For this review, use the dimensioned drawing (mm, ordinates from the lowest corner) and the shaded views. A direction names the side the tool comes from. Round coordinates to 2 decimals unless told otherwise and drop trailing zeros. Write each loop counter-clockwise with the first axis right and the second up, starting at its lowest first coordinate (ties: lowest second). Pieces come first, ordered by that corner, then holes.
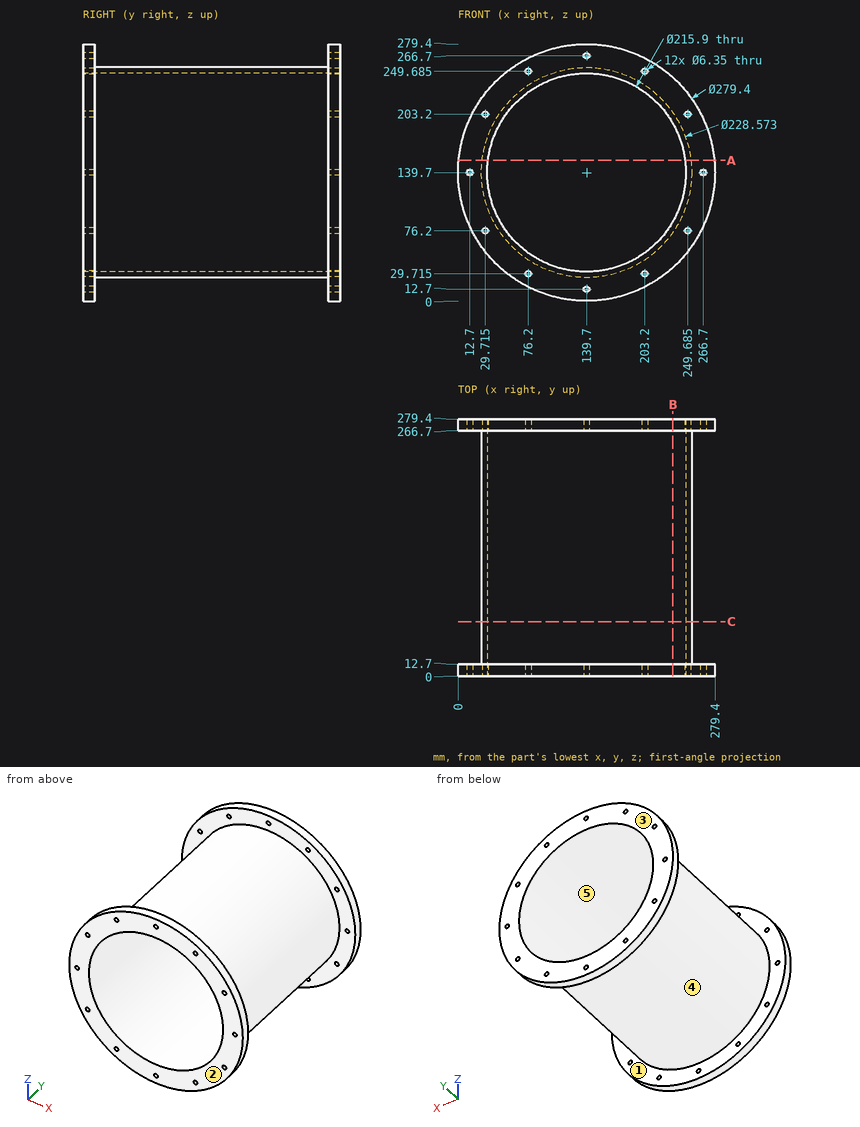
1) The part is to be moulded in two halves that separate along Z. For the marked faces 3, 4 and 5, say which applies: pulls with the +Z half, pulls with the -Z half, needs draft (parallel to the pull), parting line crosses it, or undercut.
2) Add section C-C on y = 59. State the section outline as (x, z) points.
3) For P1, Ø4, axis at x = 12.7, z = 139.7, coming from the +Y side; P2, Ø3, axis at y = 233.5, z = 200.5, coming from the +X side; P3, Ø6, axis at y = 79, z = 35, coming from the +X side; P4, Ø3, axis at x = 205.5, y = 138, coming from the -Z side, all flat-tipped, find the tip position at first contact; note any pin that passes through.
4) For line 1 along Z through (x, y) = (139, 3); line 2 along Y through (x, z) = (196, 40); line 3 along X through (y, z) = (3, 203.2) (1 decimal), list the stretches that pass through material, from the lowest coordinate up.
5) Add section B-B on x = 233.5. State the section outline as (y, z) points.
6) For the marked faces 1 and 2, list the 3-axis set-ups (+Z, -Z, +X, -X, +Y, -Y) from which the entire face can be reached by the end or side of a thin tool; tool diameter is ignored.
7) Add section A-A on z = 153. State the section outline as (x, y) points (1 decimal).
Computed:
1. face 3: needs draft
1. face 4: parting line crosses it
1. face 5: undercut
2. outline: circle Ø228.57 at (139.7, 139.7); hole circle Ø215.9 at (139.7, 139.7)
3. P1: passes through
3. P2: stops at x = 237.4
3. P3: stops at x = 191.84
3. P4: stops at z = 45.22
4. line 1: z = 0 to 9.6, 15.8 to 31.75, 247.65 to 263.6, 269.8 to 279.4
4. line 2: y = 0 to 12.7, 266.7 to 279.4
4. line 3: x = 15.3 to 26.5, 32.9 to 52.4, 227 to 246.5, 252.9 to 264.1
5. outline: (0, 36.17) - (12.7, 36.17) - (12.7, 74.41) - (266.7, 74.41) - (266.7, 36.17) - (279.4, 36.17) - (279.4, 86.27) - (0, 86.27) - close; (0, 193.13) - (279.4, 193.13) - (279.4, 243.23) - (266.7, 243.23) - (266.7, 204.99) - (12.7, 204.99) - (12.7, 243.23) - (0, 243.23) - close
6. face 1: none
6. face 2: +Z, -Z, +X, -X, -Y
7. outline: (0.6, 0) - (32.6, 0) - (32.6, 279.4) - (0.6, 279.4) - (0.6, 266.7) - (26.2, 266.7) - (26.2, 12.7) - (0.6, 12.7) - close; (246.8, 0) - (278.8, 0) - (278.8, 12.7) - (253.2, 12.7) - (253.2, 266.7) - (278.8, 266.7) - (278.8, 279.4) - (246.8, 279.4) - close
